Model file for the job. Use its own axes, mm. A direction names the side the tool comes from. Round coordinates to 2 decimals unless told otherwise and drop trailing zeros. Order: outer loops, then holes, each group sorted by start corner. A loop starts at its lowest first (then second) coordinate and runs counter-clockwise, first axis right, second up. Notation, with made-up numbers: (-32.5, -23.75) - (-13.5, -23.75) arc R16 cw to (-13.5, -0.75) - close; hole circle Ø7 at (54.5, 67). An arc over 180 degrees is marked (long way). Use one line per item in the form item = value.
Autodesk Inventor part; units mm, degrees
ref_plane "YZ Plane" through (0, 0, 0) normal (1, 0, 0) x (0, 1, 0)
ref_plane "XZ Plane" through (0, 0, 0) normal (0, 1, 0) x (-1, 0, 0)
ref_plane "XY Plane" through (0, 0, 0) normal (0, 0, 1) x (1, 0, 0)
sketch "Sketch1" plane through (0, 0, 0) normal (0, 1, 0) x (-1, 0, 0)
  line L0 (7.5, 12.5) -> (-7.5, 12.5)
  line L1 (-7.5, 12.5) -> (-7.5, -12.5)
  line L2 (-7.5, -12.5) -> (7.5, -12.5)
  line L3 (7.5, -12.5) -> (7.5, 12.5)
  point P0 (0, 0)
  dimension "d0" = 25
  dimension "d1" = 15
  dimension "d2" = 7.5
  dimension "d3" = 12.5
extrude "Extrusion1" add sketch "Sketch1" along normal blind 10
sketch "Sketch3" plane through (7.5, 0, 12.5) normal (1, 0, 0) x (0, 0, -1)
  line L0 (0, 0) -> (0, 10)
  line L1 (0, 5) -> (25, 5)
  line L2 (25, 5) -> (25, 4.2)
  line L3 (25, 4.2) -> (0, 4.2)
  line L4 (0, 4.2) -> (0, 5)
  point P0 (12.5, 0)
  dimension "d8" = 0.8
  dimension "d9" = 25
extrude "Extrusion2" cut sketch "Sketch3" against normal blind 7
sketch "Sketch4" plane through (0, 10, 0) normal (0, 1, 0) x (1, 0, 0)
  circle A0 centre (3.69, -6.15) radius 1.5316
  line L0 (-7.5, -12.5) -> (7.5, -12.5)
  line L1 (7.5, -12.5) -> (7.5, 12.5)
  circle A1 centre (-3.69, -6.15) radius 1.5367
  line L2 (-7.5, 12.5) -> (-7.5, -12.5)
  point P0 (0, 0)
  dimension "d12" = 6.35
  dimension "d13" = 3.81
  dimension "d14" = 3.0631
  dimension "d15" = 3.81
  dimension "d16" = 3.0734
  dimension "d17" = 6.35
sketch "Sketch5" plane through (0, 10, 0) normal (0, 1, 0) x (1, 0, 0)
  circle A0 centre (3.69, 6.15) radius 1.5367
  circle A1 centre (-3.69, 6.15) radius 1.5367
  line L0 (7.5, 12.5) -> (-7.5, 12.5)
  line L1 (-7.5, 12.5) -> (-7.5, -12.5)
  line L2 (7.5, -12.5) -> (7.5, 12.5)
  point P0 (0, 0)
  dimension "d18" = 6.35
  dimension "d19" = 6.35
  dimension "d20" = 3.81
  dimension "d21" = 3.81
  dimension "d22" = 3.0734
  dimension "d23" = 3.0734
ref_plane "Work Plane1" through (0, 16, 0) normal (0, 1, 0) x (1, 0, 0)
sketch "Sketch6" plane through (0, 16, 0) normal (0, 1, 0) x (1, 0, 0)
  circle A0 centre (3.69, 6.15) radius 0.254
  line L0 (7.5, 12.5) -> (-7.5, 12.5)
  line L1 (7.5, -12.5) -> (7.5, 12.5)
  point P0 (0, 0)
  dimension "d41" = 0.508
  dimension "d42" = 6.35
  dimension "d43" = 3.81
loft "Loft1" add profiles "Sketch6", "Sketch5" contours all / A0
sketch "Sketch7" plane through (0, 16, 0) normal (0, 1, 0) x (1, 0, 0)
  circle A0 centre (3.69, -6.15) radius 0.254
  line L0 (7.5, -12.5) -> (7.5, 12.5)
  line L1 (-7.5, -12.5) -> (7.5, -12.5)
  point P0 (0, 0)
  dimension "d44" = 0.508
  dimension "d45" = 3.81
  dimension "d46" = 6.35
loft "Loft2" add profiles "Sketch4", "Sketch7" contours A0 / all
sketch "Sketch10" plane through (0, 16, 0) normal (0, 1, 0) x (1, 0, 0)
  circle A0 centre (-3.69, -6.15) radius 0.254
  line L0 (-7.5, 12.5) -> (-7.5, -12.5)
  line L1 (-7.5, -12.5) -> (7.5, -12.5)
  point P0 (0, 0)
  dimension "d53" = 3.81
  dimension "d54" = 6.35
  dimension "d55" = 0.508
loft "Loft3" add profiles "Sketch4", "Sketch10" contours A1 / all
sketch "Sketch11" plane through (0, 16, 0) normal (0, 1, 0) x (1, 0, 0)
  circle A0 centre (-3.69, 6.15) radius 0.254
  line L0 (-7.5, 12.5) -> (-7.5, -12.5)
  line L1 (7.5, 12.5) -> (-7.5, 12.5)
  point P0 (0, 0)
  dimension "d60" = 0.508
  dimension "d61" = 3.81
  dimension "d62" = 6.35
loft "Loft4" add profiles "Sketch5", "Sketch11" contours A1 / all
properties part number "_3DPrint"
(1) Slice it at B-B on z = -10.25. Give the cut face in (x, y), then the cut area to 3 significant figures.
Report:
outline = (-7.5, 0) - (7.5, 0) - (7.5, 4.2) - (0.5, 4.2) - (0.5, 5) - (7.5, 5) - (7.5, 10) - (-7.5, 10) - close
area = 144 mm2
(2) Probe probe 1 along Y at (x, z) = (0.75, 11.25); probe 2 along Y at (x, z) = (-6, 3); probe 3 along X at (y, z) = (4.5, -0.25). List the from-to ranges inside material, lowest first. Write a range as [from, to].
Report:
probe_1 = [0, 4.2], [5, 10]
probe_2 = [0, 10]
probe_3 = [-7.5, 0.5]
(3) Slice it at C-C on y = 11.5. Give the cut face in (x, z), then the cut area to 3 significant figures.
Report:
outline = circle Ø2.43 at (-3.69, -6.15); circle Ø2.43 at (-3.69, 6.15); circle Ø2.43 at (3.69, -6.15); circle Ø2.42 at (3.69, 6.15)
area = 18.6 mm2
(4) Slice it at A-A on x = 6.75. Give the cut face in (y, z), then the cut area to 3 significant figures.
Report:
outline = (0, -12.5) - (4.2, -12.5) - (4.2, 12.5) - (0, 12.5) - close; (5, -12.5) - (10, -12.5) - (10, 12.5) - (5, 12.5) - close
area = 230 mm2
(5) Pull direction Z, two halves, no side cores. Call faces 1 (the face through (-7.5, 5, 0)), 2 (the face through (-3.89, 12.96, -7.03)), 3 (the face through (0, 5, 12.5)): released by +Z, released by -Z, zero draft, split by the parting line, or undercut.
Report:
face_1 = zero draft
face_2 = undercut
face_3 = released by +Z
(6) Slice it at D-D on x = -1. Give the cut face in (y, z).
Report:
outline = (0, -12.5) - (10, -12.5) - (10, 12.5) - (0, 12.5) - close
(7) Tool access for faces 4 (the face through (4, 4.2, 0)), 5 (the face through (0, 0, 0)): list every direction of +Z, -Z, +X, -X, +Y, -Y with a clear straight run to the whole face (end or side of a thin tool).
Report:
face_4 = +Z, -Z, +X
face_5 = +Z, -Z, +X, -X, -Y
(8) Pin check, flat tip, straight feed: pin 1 (1 mm diameter, centred on y = 13.5, z = -8, fed in from -X). Stop position of the tip, or through.
Report:
pin_1 = through
